Can you work these out from the drawing? Everything is in mm from the part's minimum corner. A direction names the side the tool comes from. Coordinates: 2 decimals unless noted, no trailing zeros. Loops run counter-clockwise (first coordinate to the right, second up) from the corner with the lowest first, then second, coordinate; pieces in that order, holes last.
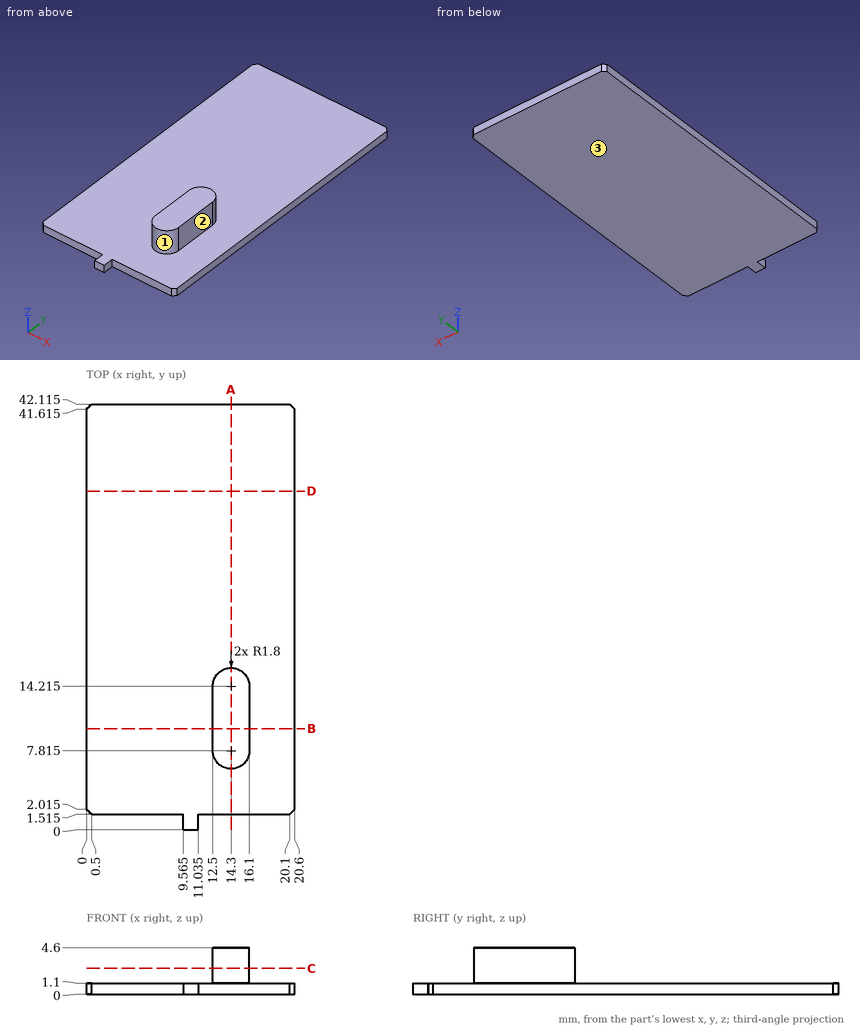
1. For pin 1 (0.6 mm diameter, centred on x = 17.5, z = 0.5, fed in from -Y) (1 decimal); pin 2 (1.7 mm diameter, centred on y = 11, z = 3.5, fed in from +X); pin 3 (1.7 mm diameter, centred on y = 11, z = 2, fed in from -X), each with a flat end and sliding along its axis, tell me the tip position at first contact or that it passes through.
2. I want a section at C-C (z = 2.55). Please give me the cut outline in (x, y) (1 decimal), then the cut area to 3 significant figures.
3. I need wall thicknesses on line 1 along Z through (x, y) = (12, 23.5); line 2 along X through (y, z) = (8.5, 3.1); line 3 along Y through (x, z) = (14.25, 3.1) (1 decimal). Which ranges of each line are inside material? Lowest first, please.
4. I want a section at B-B (y = 10). Please give me the cut outline in (x, z).
5. On a 3-axis mill with a long thin cutter (end or side, diameter ignored), from which of +Z, -Z, +X, -X, +Y, -Y can I reach the whole of each face in a straight line? I mean the marked faces 1, 2 and 3. Say none if no direction works.
6. I want a section at A-A (x = 14.3). Please give me the cut outline in (y, z) (1 decimal).
7. I want a section at D-D (y = 33.5). Please give me the cut outline in (x, z).
Response values:
1. pin 1: stops at y = 1.5
1. pin 2: stops at x = 16.1
1. pin 3: stops at x = 12.5
2. outline: (12.5, 7.8) arc R1.8 ccw to (16.1, 7.8) - (16.1, 14.2) arc R1.8 ccw to (12.5, 14.2) - close
2. area: 33.2 mm2
3. line 1: z = 0 to 1.1
3. line 2: x = 12.5 to 16.1
3. line 3: y = 6 to 16
4. outline: (0, 0) - (20.6, 0) - (20.6, 1.1) - (16.1, 1.1) - (16.1, 4.6) - (12.5, 4.6) - (12.5, 1.1) - (0, 1.1) - close
5. face 1: +Z, -Y
5. face 2: +Z, +X, +Y, -Y
5. face 3: -Z, +X, -X, +Y, -Y
6. outline: (1.5, 0) - (42.1, 0) - (42.1, 1.1) - (16, 1.1) - (16, 4.6) - (6, 4.6) - (6, 1.1) - (1.5, 1.1) - close
7. outline: (0, 0) - (20.6, 0) - (20.6, 1.1) - (0, 1.1) - close
